from build123d import *

# Parameters (mm, degrees)
SKETCH_1_W      = 25
SKETCH_1_H      = 11
EXTRUDE_1_DEPTH = 3
CHAMFER_3_SIZE  = 2


with BuildPart() as part:
    # Эскиз1 → Вытянуть1 (new body)
    with BuildSketch(Plane.XY):
        with Locations((-0.5, 0)):
            Rectangle(SKETCH_1_W, SKETCH_1_H)
    extrude(amount=EXTRUDE_1_DEPTH)

    # Фаска3
    chamfer_3_edges = [part.edges().sort_by_distance(p)[0] for p in [
        (-0.5, -5.5, 3),
    ]]
    chamfer(chamfer_3_edges, length=CHAMFER_3_SIZE)


solid = part.part
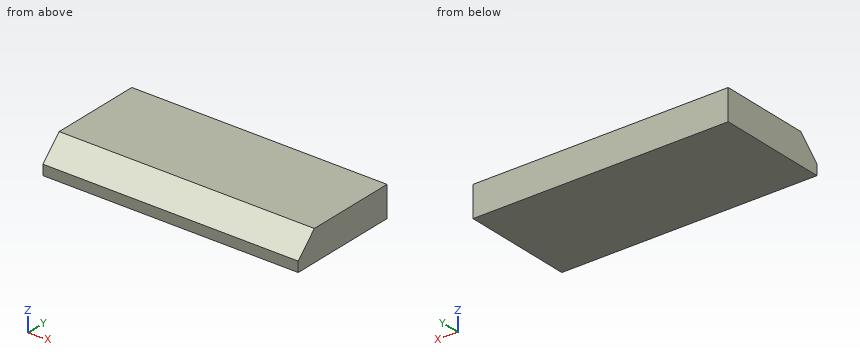
Read the model definition and answer for the solid it produces. Units are mm, in the model's axes. Coordinates: 2 decimals unless noted, no trailing zeros. Loops run counter-clockwise (first coordinate to the right, second up) from the corner with the lowest first, then second, coordinate; pieces in that order, holes last.
Q1. The part is cut by section B-B on z = 1.9. Write down the section's boundary in (x, y), and give its area (4 significant figures).
Q2. The part is cut by section A-A on x = -0.5. Write down the section's boundary in (y, z).
Q3. Consider probe 1 along Y at (x, z) = (-0.5, 2.7); probe 2 along Y at (x, z) = (-8, 1.2); probe 3 along Z at (x, y) = (0.25, -4.75). Determine where each line is inside the solid, lowest interval first.
Results below:
1. outline: (-13, -4.6) - (12, -4.6) - (12, 5.5) - (-13, 5.5) - close
1. area: 252.5 mm2
2. outline: (-5.5, 0) - (5.5, 0) - (5.5, 3) - (-3.5, 3) - (-5.5, 1) - close
3. probe 1: y = -3.8 to 5.5
3. probe 2: y = -5.3 to 5.5
3. probe 3: z = 0 to 1.75
